Geometry check sheet. Reference: the model listing, model coordinates, mm. Round coordinates to 2 decimals unless told otherwise and drop trailing zeros. Write each loop counter-clockwise with the first axis right and the second up, starting at its lowest first coordinate (ties: lowest second). Pieces come first, ordered by that corner, then holes. Notation, with made-up numbers: M 67,13.25 L 84,13.25 A22 cw 84,52.25 Z; hole C -34.75,-27 d4. An arc over 180 degrees is marked long. Put each result on its own line as item: value. Start each with the question number.
(1) Mould release check, pull along X, two halves, no side actions. Record for faces 1 (the flat face through (-1, 13, -60.008)), 2 (the flat face through (60.008, 13, 1)), 3 (the cylindrical face through (54.21, 12.52, -54.34)), 4 (the cylindrical face through (2.58, 12.88, -58.68)): pulls with the +X half, pulls with the -X half, needs draft (parallel to the pull), parting line crosses it, or undercut.
(2) Section check A-A on x = 0. Record the cut outline in (y, z).
(3) Material ranges on probe 1 along X at (y, z) = (2, 30); probe 2 along X at (y, z) = (5.5, 0); probe 3 along Z at (x, y) = (1.5, 7.25), recorded low to high.
(4) Section check C-C on y = 16. Record the cut outline in (x, z) (1 decimal), then the cut area to 3 significant figures.
(5) Section check B-B on z = 0. Record the cut outline in (x, y).
from build123d import *

# Parameters (mm, degrees)
SKETCH1_W           = 120.015
SKETCH1_H           = 120.015
SKETCH1_R           = 2.2225
BOSS_EXTRUDE1_DEPTH = 25.4
SKETCH2_R           = 58.7375
CUT_EXTRUDE1_DEPTH  = 89.583068995


with BuildPart() as part:
    # Sketch1 → Boss-Extrude1 (new body)
    with BuildSketch(Plane(origin=(0, 0, 0), x_dir=(1, 0, 0), z_dir=(0, 1, 0))):
        Rectangle(SKETCH1_W, SKETCH1_H)
        with Locations(Location((-52.705, 52.705, 0), (0, 0, 270))):
            Circle(SKETCH1_R, mode=Mode.SUBTRACT)
        with Locations(Location((52.705, -52.705, 0), (0, 0, 90))):
            Circle(SKETCH1_R, mode=Mode.SUBTRACT)
        with Locations(Location((52.705, 52.705, 0), (0, 0, 270))):
            Circle(SKETCH1_R, mode=Mode.SUBTRACT)
        with Locations(Location((-52.705, -52.705, 0), (0, 0, 90))):
            Circle(SKETCH1_R, mode=Mode.SUBTRACT)
    extrude(amount=BOSS_EXTRUDE1_DEPTH)

    # Sketch2 → Cut-Extrude1 (cut, through all)
    with BuildSketch(Plane(origin=(0, 25.4, 0), x_dir=(1, 0, 0), z_dir=(0, 1, 0))):
        with Locations(Location((0, 0, 0), (0, 0, 270))):
            Circle(SKETCH2_R)
    extrude(amount=-CUT_EXTRUDE1_DEPTH, mode=Mode.SUBTRACT)


solid = part.part
Answers follow:
1. face 1: needs draft
1. face 2: pulls with the +X half
1. face 3: undercut
1. face 4: undercut
2. outline: M 0,-60.01 L 25.4,-60.01 L 25.4,-58.74 L 0,-58.74 Z; M 0,58.74 L 25.4,58.74 L 25.4,60.01 L 0,60.01 Z
3. probe 1: x = -60.01 to -50.5, 50.5 to 60.01
3. probe 2: x = -60.01 to -58.74, 58.74 to 60.01
3. probe 3: z = -60.01 to -58.72, 58.72 to 60.01
4. outline: M -60,-60 L 60,-60 L 60,60 L -60,60 Z; hole C 0,0 d117.5; hole C -52.7,-52.7 d4.4; hole C -52.7,52.7 d4.4; hole C 52.7,-52.7 d4.4; hole C 52.7,52.7 d4.4
4. area: 3,500 mm^2
5. outline: M -60.01,0 L -58.74,0 L -58.74,25.4 L -60.01,25.4 Z; M 58.74,0 L 60.01,0 L 60.01,25.4 L 58.74,25.4 Z
